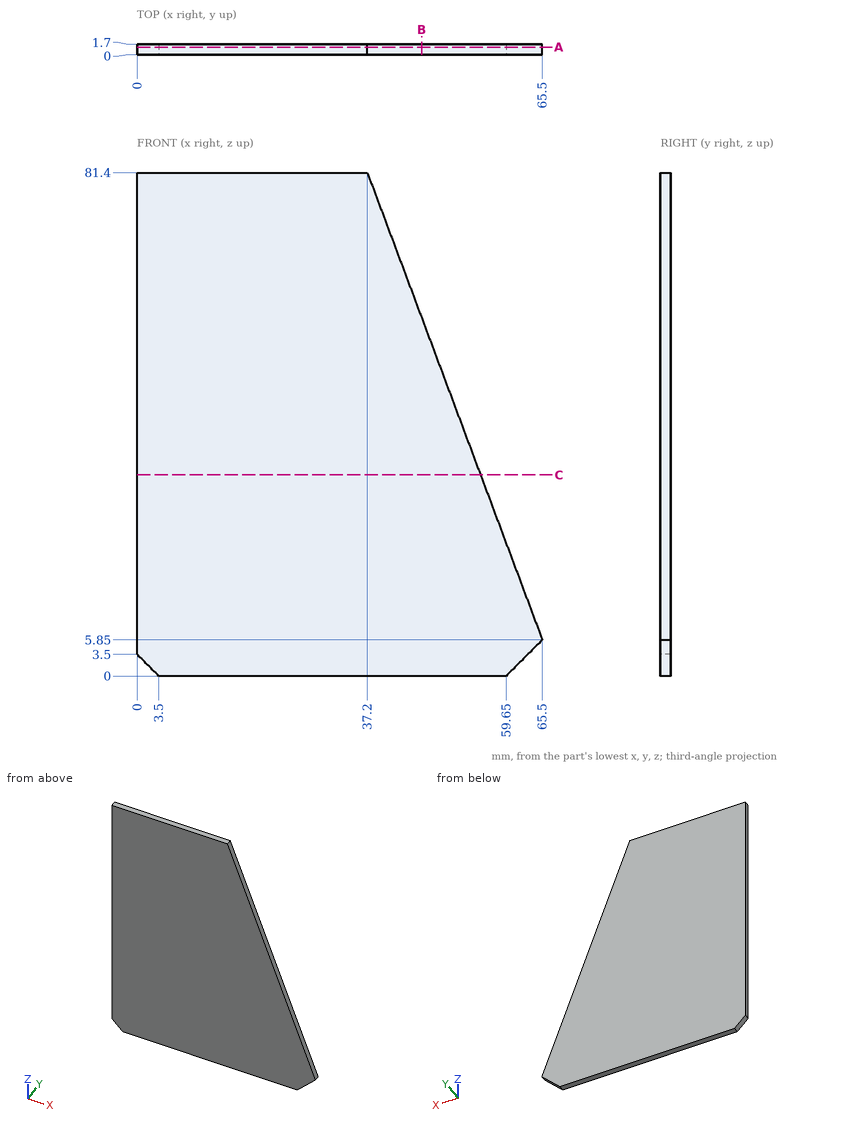
Drawing for the job (mm, zero at the part's lowest x, y, z). Coordinates: 2 decimals unless noted, no trailing zeros. Order: outer loops, then holes, each group sorted by start corner. A loop starts at its lowest first (then second) coordinate and runs counter-clockwise, first axis right, second up. Notation, with made-up numbers: (-25.5, -0.5) -> (15.5, -0.5) arc R10 ccw to (15.5, 6.5) -> close; hole circle Ø1 at (-39.75, 68.5). An arc over 180 degrees is marked (long way). One line per item, written item: value.
(1) Slice it at B-B, the plane x = 46. List the corners of the cut face in (y, z).
Checked values:
outline: (0, 0) -> (1.7, 0) -> (1.7, 57.91) -> (0, 57.91) -> close
(2) Slice it at C-C, the plane z = 32.5. List the corners of the cut face in (x, y), plus the area to 3 significant figures.
Checked values:
outline: (0, 0) -> (55.52, 0) -> (55.52, 1.7) -> (0, 1.7) -> close
area: 94.4 mm2
(3) Slice it at A-A, the plane y = 1.2. List the corners of the cut face in (x, z).
Checked values:
outline: (0, 3.5) -> (3.5, 0) -> (59.65, 0) -> (65.5, 5.85) -> (37.2, 81.4) -> (0, 81.4) -> close
(4) Probe line 1 (X direction, y = 1, z = 20.5); line 2 (X direction, y = 1.1, z = 60). List the from-to ranges inside material, lowest first. Write a range as [from, to].
Checked values:
line 1: [0, 60.01]
line 2: [0, 45.22]
